Verification items for the finished model (mm, model axes). A direction names the side the tool comes from. Coordinates: 2 decimals unless noted, no trailing zeros. Answer in a Markdown table with one row per item.
from build123d import *

# Parameters (mm, degrees)
SZKIC1_W                    = 4
SZKIC1_H                    = 4
DODANIE_WYCI_GNI_CIE1_DEPTH = 34
SZKIC2_W                    = 4
SZKIC2_H                    = 4
DODANIE_WYCI_GNI_CIE2_DEPTH = 50
SZKIC3_W                    = 4
SZKIC3_H                    = 4
DODANIE_WYCI_GNI_CIE3_DEPTH = 73
SZKIC4_W                    = 4
SZKIC4_H                    = 4
DODANIE_WYCI_GNI_CIE4_DEPTH = 50
SZKIC5_W                    = 4
SZKIC5_H                    = 4
DODANIE_WYCI_GNI_CIE5_DEPTH = 34
ZAOKR_GLENIE1_R             = 2


with BuildPart() as part:
    # Szkic1 → Dodanie-wyciągnięcie1 (new body)
    with BuildSketch(Plane(origin=(0, 0, 0), x_dir=(1, 0, 0), z_dir=(0, 1, 0))):
        Rectangle(SZKIC1_W, SZKIC1_H)
    extrude(amount=DODANIE_WYCI_GNI_CIE1_DEPTH)

    # Szkic2 → Dodanie-wyciągnięcie2 (add)
    with BuildSketch(Plane.XY.offset(2)):
        with Locations((0, 32)):
            Rectangle(SZKIC2_W, SZKIC2_H)
    extrude(amount=DODANIE_WYCI_GNI_CIE2_DEPTH)

    # Szkic3 → Dodanie-wyciągnięcie3 (add)
    with BuildSketch(Plane.XZ.offset(-30)):
        with Locations((0, 50)):
            Rectangle(SZKIC3_W, SZKIC3_H)
    extrude(amount=DODANIE_WYCI_GNI_CIE3_DEPTH)

    # Szkic4 → Dodanie-wyciągnięcie4 (add)
    with BuildSketch(Plane(origin=(0, 0, 48), x_dir=(-1, 0, 0), z_dir=(0, 0, -1))):
        with Locations((0, -41)):
            Rectangle(SZKIC4_W, SZKIC4_H)
    extrude(amount=DODANIE_WYCI_GNI_CIE4_DEPTH)

    # Szkic5 → Dodanie-wyciągnięcie5 (add)
    with BuildSketch(Plane(origin=(0, -39, 0), x_dir=(1, 0, 0), z_dir=(0, 1, 0))):
        Rectangle(SZKIC5_W, SZKIC5_H)
    extrude(amount=DODANIE_WYCI_GNI_CIE5_DEPTH)

    # Zaokrąglenie1
    zaokr_glenie1_edges = [part.edges().sort_by_distance(p)[0] for p in [
        (2, 34, 25),
        (0, 34, -2),
        (2, 15, 2),
        (-2, 15, 2),
        (0, 30, 2),
        (-2, -4.5, 52),
        (2, -4.5, 52),
        (0, 34, 52),
        (2, 30, 25),
        (-2, 30, 25),
        (0, 30, 48),
        (-2, -43, 25),
        (2, -43, 25),
        (0, -43, 52),
        (2, -4.5, 48),
        (-2, -4.5, 48),
        (-2, 34, 25),
        (0, -39, 48),
        (-2, -24, -2),
        (2, -24, -2),
        (0, -43, -2),
        (0, 0, -2),
        (2, 0, 0),
        (2, -39, 25),
        (-2, -39, 25),
        (0, 0, 2),
        (2, -22, 2),
        (0, -39, 2),
        (-2, -22, 2),
        (2, -5, 0),
        (0, -5, -2),
        (-2, -5, 0),
        (0, -5, 2),
        (-2, 0, 0),
        (-2, 17, -2),
        (2, 17, -2),
    ]]
    fillet(zaokr_glenie1_edges, radius=ZAOKR_GLENIE1_R - 0.0001)  # a hair under: the kernel refuses the full size


solid = part.part
1) Depth check by flat-ended pin: pin 1 (2 mm diameter, centred on x = 1.5, y = -32.5, fed in from +Z); pin 2 (2 mm diameter, centred on x = -0.5, z = 34.5, fed in from +Y). Enter the tip coordinate at first touch or a pass-through.
Response values:
| item | result |
|---|---|
| pin 1 | stops at z = 51.94 |
| pin 2 | stops at y = 34 |
2) Thickness scan on L1, parallel to Z at x = -0.05, y = -35.5; L2, parallel to Y at x = 0, z = 27; L3, parallel to Z at x = 1.7, y = 8.5. Record the ranges inside material, lowest first. Write a range as [from, to].
Response values:
| item | result |
|---|---|
| L1 | z = [-2, 2], [48, 52] |
| L2 | y = [-43, -39], [30, 34] |
| L3 | z = [-1.05, 1.05], [48.95, 51.05] |
3) Tool access check on faces 1 (the face through (-1.43, -21.79, 1.4)), 2 (the face through (1.43, 30.6, 25.29)), 3 (the face through (-1.43, -42.4, 24.65)). Record the directions out of +Z, -Z, +X, -X, +Y, -Y that give a thin tool (end or side, any length) a straight path to the whole face; none if there is none.
Response values:
| item | result |
|---|---|
| face 1 | -X |
| face 2 | +X |
| face 3 | +Z, -Z, -X, -Y |
4) Release check for a two-part mould opening along Y. For faces 4 (the face through (1.43, -42.4, 24.65)), 5 (the face through (1.4, -39.57, 24.71)), 6 (the face through (-1.43, -3.99, 51.4)), 7 (the face through (1.43, 15.18, 1.4)) record: +Y half, -Y half, draft (parallel to the pull), parting line (faces both ways), or undercut.
Response values:
| item | result |
|---|---|
| face 4 | -Y half |
| face 5 | undercut |
| face 6 | draft |
| face 7 | undercut |
